```python
from build123d import *

# Parameters (mm, degrees)
F0_W     = 26
F0_H     = 29
F0_R     = 2.5
F1_DEPTH = 16
F2_R     = 5
F3_DEPTH = 60
F4_W     = 10.5
F4_H     = 5
F5_DEPTH = 60
F6_R     = 1


with BuildPart() as f1:
    # F0 (on Top) → F1 (new body)
    with BuildSketch(Plane.XY):
        Rectangle(F0_W, F0_H)
        with Locations((-6.5, -8)):
            Circle(F0_R, mode=Mode.SUBTRACT)
        with Locations((-6.5, 8)):
            Circle(F0_R, mode=Mode.SUBTRACT)
    extrude(amount=F1_DEPTH)

    # F2 (on face) → F3 (cut)
    with BuildSketch(Plane.XZ.offset(14.5)):
        with Locations((3.5, 7.2)):
            Circle(F2_R)
    extrude(amount=-F3_DEPTH, mode=Mode.SUBTRACT)

    # F4 (on face) → F5 (cut)
    with BuildSketch(Plane.XZ.offset(14.5)):
        with Locations((7.75, 2.5)):
            Rectangle(F4_W, F4_H)
    extrude(amount=-F5_DEPTH, mode=Mode.SUBTRACT)

    # F6
    f6_edges = [f1.edges().sort_by_distance(p)[0] for p in [
        (0, -14.5, 16),
        (-13, 0, 16),
        (13, 0, 16),
        (0, 14.5, 16),
        (7.989989, 0, 5),
        (2.5, 0, 2.301021),
        (1.29407, -14.5, 11.687078),
        (1.29407, 14.5, 11.687078),
    ]]
    fillet(f6_edges, radius=F6_R)


solid = f1.part
```
Input: part model. Units: mm. Frame: model coordinates. A direction names the side the tool comes from. Round coordinates to 2 decimals unless told otherwise and drop trailing zeros. Loops run counter-clockwise (first coordinate to the right, second up) from the corner with the lowest first, then second, coordinate; pieces in that order, holes last.
1) Section query B-B on z = 7.2. Return the cut outline in (x, y), plus the area to 3 significant figures.
Ans:
outline: (-13, -14.5) - (-2.5, -14.5) arc R1 ccw to (-1.5, -13.5) - (-1.5, 13.5) arc R1 ccw to (-2.5, 14.5) - (-13, 14.5) - close; (8.5, -13.5) arc R1 ccw to (9.5, -14.5) - (13, -14.5) - (13, 14.5) - (9.5, 14.5) arc R1 ccw to (8.5, 13.5) - close; hole circle Ø5 at (-6.5, -8); hole circle Ø5 at (-6.5, 8)
area: 424 mm2
2) Section query C-C on y = -8. Return the cut outline in (x, z).
Ans:
outline: (-13, 0) - (-9, 0) - (-9, 16) - (-12, 16) arc R1 ccw to (-13, 15) - close; (-4, 0) - (2.5, 0) - (2.5, 1.54) arc R1 ccw to (1.83, 2.49) arc R5 cw (long way) to (8.4, 6.2) arc R1 ccw to (9.38, 5) - (13, 5) - (13, 15) arc R1 ccw to (12, 16) - (-4, 16) - close
3) Material intervals for line 1 (Y direction, x = -6.5, z = 6.75); line 2 (Y direction, x = -4.75, z = 4.25); line 3 (X direction, y = -9.25, z = 11.25), sorted ascending.
Ans:
line 1: y = -14.5 to -10.5, -5.5 to 5.5, 10.5 to 14.5
line 2: y = -14.5 to -9.79, -6.21 to 6.21, 9.79 to 14.5
line 3: x = -13 to -8.67, -4.33 to 0.57, 6.43 to 13
4) Section query A-A on x = -6.5. Return the cut outline in (y, z), plus the area to 3 significant figures.
Ans:
outline: (-14.5, 0) - (-10.5, 0) - (-10.5, 16) - (-13.5, 16) arc R1 ccw to (-14.5, 15) - close; (-5.5, 0) - (5.5, 0) - (5.5, 16) - (-5.5, 16) - close; (10.5, 0) - (14.5, 0) - (14.5, 15) arc R1 ccw to (13.5, 16) - (10.5, 16) - close
area: 304 mm2
5) Pin query (flat end, axial travel): pin 1 (1.1 mm diameter, centred on x = 12, y = -1, fed in from -Z); pin 2 (3 mm diameter, centred on x = -6.5, y = 8, fed in from -Z); pin 3 (0.5 mm diameter, centred on y = -2.5, z = 0.5, fed in from +X); pin 4 (4 mm diameter, centred on x = 5, y = 6.5, fed in from -Z). Return the tip coordinate at first contact, or that it passes through.
Ans:
pin 1: stops at z = 5
pin 2: passes through
pin 3: stops at x = 2.5
pin 4: stops at z = 10.77
6) Section query D-D on x = 10.5. Return the cut outline in (y, z), plus the area to 3 significant figures.
Ans:
outline: (-14.5, 5) - (14.5, 5) - (14.5, 15) arc R1 ccw to (13.5, 16) - (-13.5, 16) arc R1 ccw to (-14.5, 15) - close
area: 319 mm2
7) Pull-direction query (Y, two-part tool) for faces 4 (the cylindrical face through (0.182, -14.199, 15.715)), 5 (the cylindrical face through (-5, -10, 8)), 6 (the flat face through (-5, 0, 0)); classes: released by +Y, released by -Y, zero draft, split by the parting line, or undercut.
Ans:
face 4: released by -Y
face 5: undercut
face 6: zero draft
8) Set-up query: faces 1 (the flat face through (-3, -14.5, 9)), 2 (the cylindrical face through (2.31, -0.2, 2.13)), 3 (the flat face through (11, 0, 5)). Return all of +Z, -Z, +X, -X, +Y, -Y with unobstructed straight access to the full face (end or side cutting, diameter ignored); none if empty.
Ans:
face 1: +Z, -Z, +X, -X, -Y
face 2: +X, +Y, -Y
face 3: -Z, +X, +Y, -Y
